```python
from build123d import *

# Parameters (mm, degrees)
BOSS_EXTRUDE1_DEPTH       = 9.2964
BOSS_EXTRUDE2_DEPTH       = 16.002
BOSS_EXTRUDE3_DEPTH       = 10.795
SKETCH4_R                 = 11
BOSS_EXTRUDE4_DEPTH       = 1.5
SKETCH5_R                 = 2.54
BOSS_EXTRUDE5_DEPTH       = 24
F_2_CLEARANCE_HOLE1_D     = 2.5
F_2_CLEARANCE_HOLE1_DEPTH = 6
F_2_CLEARANCE_HOLE1_TIP   = 0.751075774
FILLET1_R                 = 2


with BuildPart() as part:
    # Sketch1 → Boss-Extrude1 (new body)
    with BuildSketch(Plane.XY.offset(8)):
        Polygon((-21, 15), (-21, -15), (-15, -21), (15, -21), (21, -15), (21, 15), (15, 21), (-15, 21), align=None)
    extrude(amount=-BOSS_EXTRUDE1_DEPTH)

    # Sketch2 → Boss-Extrude2 (add)
    with BuildSketch(Plane(origin=(0, 0, -1.2964), x_dir=(-1, 0, 0), z_dir=(0, 0, -1))):
        with BuildLine():
            Line((-10.735086841, 20.75), (10.735086841, 20.75))
            ThreePointArc((10.735086841, 20.75), (11.503053413, 20.366719307), (12.171572875, 19.828427125))
            Line((12.171572875, 19.828427125), (19.828427125, 12.171572875))
            ThreePointArc((19.828427125, 12.171572875), (20.366719307, 11.503053413), (20.75, 10.735086841))
            Line((20.75, 10.735086841), (20.75, -10.735086841))
            ThreePointArc((20.75, -10.735086841), (20.366719307, -11.503053413), (19.828427125, -12.171572875))
            Line((19.828427125, -12.171572875), (12.171572875, -19.828427125))
            ThreePointArc((12.171572875, -19.828427125), (11.503053413, -20.366719307), (10.735086841, -20.75))
            Line((10.735086841, -20.75), (-10.735086841, -20.75))
            ThreePointArc((-10.735086841, -20.75), (-11.503053413, -20.366719307), (-12.171572875, -19.828427125))
            Line((-12.171572875, -19.828427125), (-19.828427125, -12.171572875))
            ThreePointArc((-19.828427125, -12.171572875), (-20.366719307, -11.503053413), (-20.75, -10.735086841))
            Line((-20.75, -10.735086841), (-20.75, 10.735086841))
            ThreePointArc((-20.75, 10.735086841), (-20.366719307, 11.503053413), (-19.828427125, 12.171572875))
            Line((-19.828427125, 12.171572875), (-12.171572875, 19.828427125))
            ThreePointArc((-12.171572875, 19.828427125), (-11.503053413, 20.366719307), (-10.735086841, 20.75))
        make_face()
    extrude(amount=BOSS_EXTRUDE2_DEPTH)

    # Sketch3 → Boss-Extrude3 (add)
    with BuildSketch(Plane.XY.offset(-16.256)):
        Polygon((-21, 15), (-21, -15), (-15, -21), (15, -21), (21, -15), (21, 15), (15, 21), (-15, 21), align=None)
    extrude(amount=-BOSS_EXTRUDE3_DEPTH)

    # Sketch4 → Boss-Extrude4 (add)
    with BuildSketch(Plane.XY.offset(8)):
        Circle(SKETCH4_R)
    extrude(amount=BOSS_EXTRUDE4_DEPTH)

    # Sketch5 → Boss-Extrude5 (add)
    with BuildSketch(Plane.XY.offset(9.5)):
        Circle(SKETCH5_R)
    extrude(amount=BOSS_EXTRUDE5_DEPTH)

    # #2 Clearance Hole1
    with Locations(Plane.XY.offset(8)):
        with Locations((-15.5, 15.5), (15.5, 15.5), (-15.5, -15.5), (15.5, -15.5)):
            Hole(F_2_CLEARANCE_HOLE1_D / 2, depth=F_2_CLEARANCE_HOLE1_DEPTH)
            with Locations((0, 0, -(F_2_CLEARANCE_HOLE1_DEPTH + F_2_CLEARANCE_HOLE1_TIP / 2))):  # 118° drill point
                Cone(0, F_2_CLEARANCE_HOLE1_D / 2, F_2_CLEARANCE_HOLE1_TIP, mode=Mode.SUBTRACT)

    # Fillet1
    fillet1_edges = [part.edges().sort_by_distance(p)[0] for p in [
        (-15, 21, 3.3518),
        (15, 21, 3.3518),
        (21, 15, 3.3518),
        (21, -15, 3.3518),
        (15, -21, 3.3518),
        (-15, -21, 3.3518),
        (-21, -15, 3.3518),
        (-21, 15, 3.3518),
        (-21, 15, -21.6535),
        (-15, 21, -21.6535),
        (15, 21, -21.6535),
        (21, 15, -21.6535),
        (21, -15, -21.6535),
        (15, -21, -21.6535),
        (-15, -21, -21.6535),
        (-21, -15, -21.6535),
    ]]
    fillet(fillet1_edges, radius=FILLET1_R)


solid = part.part
```
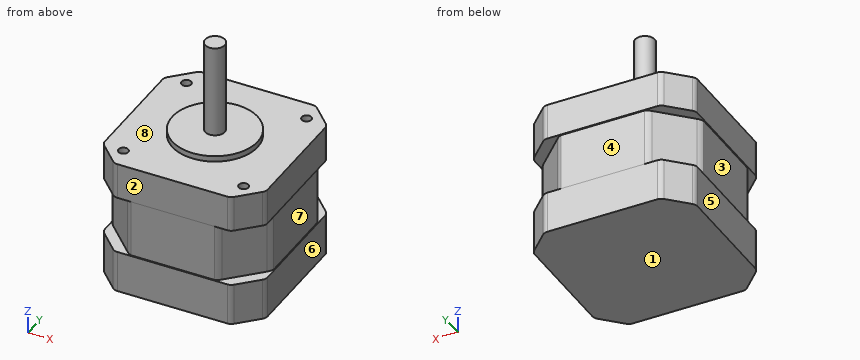
Model file for the job. Use its own axes, mm. Face numbers are marked on the shaded views. A direction names the side the tool comes from. Give positions to 0.01 mm unless a question says otherwise; leave off trailing zeros. Order: outer loops, then holes, each group sorted by start corner. A loop starts at its lowest first (then second) coordinate and runs counter-clockwise, first axis right, second up.
1) Wall check: probe 1 along Z at (x, y) = (19.5, -15); probe 2 along Y at (x, z) = (15, 3); probe 3 along Y at (x, z) = (-15.5, 6.5). Give the ranges that are in metal, low to high.
2) Saw through at D-D, the plane y = -17.5. Write the cut outline in (x, z), then the cut area to 3 significant figures.
3) Mould opens along Z. For the marked faces 1, 2 and 3 say: +Z half, -Z half, draft (parallel to the pull), parting line (faces both ways), or undercut.
4) Saw through at A-A, the plane z = -5. Write the cut outline in (x, y), then the cut area to 3 significant figures.
5) Pin check, flat tips, straight feed: pin 1 (4.5 mm diameter, centred on x = 1, z = -9, fed in from -Y); pin 2 (3 mm diameter, centred on x = -15.5, y = -15.5, fed in from +Z); pin 3 (12.5 mm diameter, centred on x = -4, y = 9, fed in from +Z). Stop position of each tip, or through.
6) Saw through at B-B, the plane y = 0. Write the cut outline in (x, z), then the cut area to 3 significant figures.
7) 3-axis set-ups, long thin cutter, end or side, ignore diameter. For the marked faces 4, 5, 6, 7 and 8: which of +Z, -Z, +X, -X, +Y, -Y reach the whole face in a straight line?
Computed:
1. probe 1: z = -27.05 to -16.26, -1.3 to 8
1. probe 2: y = -20.82 to -16.65, -14.35 to 14.35, 16.65 to 20.82
1. probe 3: y = -20.5 to -16.75, -14.25 to 14.25, 16.75 to 20.5
2. outline: (-18.5, -27.05) - (18.5, -27.05) - (18.5, -16.26) - (14.5, -16.26) - (14.5, -1.3) - (18.5, -1.3) - (18.5, 8) - (-18.5, 8) - (-18.5, -1.3) - (-14.5, -1.3) - (-14.5, -16.26) - (-18.5, -16.26) - close
2. area: 1,180 mm2
3. face 1: -Z half
3. face 2: draft
3. face 3: undercut
4. outline: (-20.75, -10.74) arc R4 ccw to (-19.83, -12.17) - (-12.17, -19.83) arc R4 ccw to (-10.74, -20.75) - (10.74, -20.75) arc R4 ccw to (12.17, -19.83) - (19.83, -12.17) arc R4 ccw to (20.75, -10.74) - (20.75, 10.74) arc R4 ccw to (19.83, 12.17) - (12.17, 19.83) arc R4 ccw to (10.74, 20.75) - (-10.74, 20.75) arc R4 ccw to (-12.17, 19.83) - (-19.83, 12.17) arc R4 ccw to (-20.75, 10.74) - close
4. area: 1,540 mm2
5. pin 1: stops at y = -20.75
5. pin 2: stops at z = 8
5. pin 3: stops at z = 9.5
6. outline: (-21, -27.05) - (21, -27.05) - (21, -16.26) - (20.75, -16.26) - (20.75, -1.3) - (21, -1.3) - (21, 8) - (11, 8) - (11, 9.5) - (2.54, 9.5) - (2.54, 33.5) - (-2.54, 33.5) - (-2.54, 9.5) - (-11, 9.5) - (-11, 8) - (-21, 8) - (-21, -1.3) - (-20.75, -1.3) - (-20.75, -16.26) - (-21, -16.26) - close
6. area: 1,620 mm2
7. face 4: +X, -X, +Y
7. face 5: +Z, -Z, -X, +Y, -Y
7. face 6: +Z, -Z, +X, +Y, -Y
7. face 7: +X, +Y, -Y
7. face 8: +Z
